Solid Edge part; units mm, degrees
sketch "Sketch1" plane through (0, 0, 0) normal (0, 0, 1) x (1, 0, 0)
  circle A0 centre (9.675, 10) radius 5
  circle A1 centre (9.675, 50) radius 5
  circle A2 centre (9.675, 90) radius 5
  circle A3 centre (70.325, 50) radius 5
  circle A4 centre (70.325, 90) radius 5
  circle A5 centre (70.325, 10) radius 5
  line L0 (0, 0) -> (80, 0)
  line L1 (80, 0) -> (80, 100)
  line L2 (0, 100) -> (80, 100)
  line L3 (0, 100) -> (0, 0)
extrude "Protrusion1" add sketch "Sketch1" along normal blind 10
sketch "Sketch2" plane through (40, 50, 10) normal (0, 0, 1) x (0, 1, 0)
  line L0 (-50, 20) -> (50, 20)
  line L1 (50, 20) -> (50, -20)
  line L2 (50, -20) -> (-50, -20)
  line L3 (-50, -20) -> (-50, 20)
extrude "ExtrudedProtrusion_2" add sketch "Sketch2" along normal blind 10
sketch "Sketch3" plane through (40, 50, 10) normal (0, 0, 1) x (0, 1, 0)
  circle A0 centre (0, 0) radius 12.5
extrude "ExtrudedCutout_1" cut sketch "Sketch3" along normal blind 10
sketch "Sketch4" plane through (40, 0, 10) normal (0, -1, 0) x (1, 0, 0)
  line L0 (20, 8) -> (20, 35)
  line L1 (-20, 35) -> (-20, 8)
  line L2 (-20, 8) -> (20, 8)
  arc A0 (-20, 35) -> (20, 35) centre (0, 35) cw
  circle A1 centre (0, 35) radius 10
extrude "ExtrudedCutout_6" cut sketch "Sketch4" against normal blind 10
sketch "Sketch5" plane through (40, 0, 10) normal (0, -1, 0) x (1, 0, 0)
  line L0 (20, 8) -> (20, 35)
  line L1 (-20, 35) -> (-20, 8)
  line L2 (-20, 8) -> (20, 8)
  arc A0 (-20, 35) -> (20, 35) centre (0, 35) cw
  circle A1 centre (0, 35) radius 10
extrude "ExtrudedProtrusion_3" add sketch "Sketch5" against normal blind 10
sketch "Sketch6" plane through (40, 0, 10) normal (0, -1, 0) x (1, 0, 0)
  circle A0 centre (0, 35) radius 17.5
  circle A1 centre (0, 35) radius 10
extrude "ExtrudedProtrusion_4" add sketch "Sketch6" along normal blind 3
mirror "Mirror1" about plane through (0, 50, 0) normal (0, -1, 0) of "ExtrudedProtrusion_3"
mirror "Mirror2" about plane through (0, 50, 0) normal (0, -1, 0) of "ExtrudedProtrusion_4"
sketch "Sketch7" plane through (40, 50, 10) normal (0, 0, 1) x (0, 1, 0)
  circle A0 centre (0, 0) radius 12.5
extrude "ExtrudedCutout_7" cut sketch "Sketch7" against normal blind 100
Work out the finished part from the listing and answer in its coordinate system (mm). A direction names the side the tool comes from. Give positions to 0.01 mm unless a question says otherwise; leave off trailing zeros. Loops run counter-clockwise (first coordinate to the right, second up) from the corner with the lowest first, then second, coordinate; pieces in that order, holes last. Notation, with made-up numbers: M 69.25,66 L 78.25,66 A22 cw 78.25,101 Z; hole C -21,10.25 d11. An arc over 180 degrees is marked long. One line per item, written item: value. Start each with the question number.
1. Determine the mould class of faces 5 (the face through (8.59, 94.88, 4.93)), 6 (the face through (32, 103, 53)), 7 (the face through (40, 5, 65)) for opening direction Y: released by +Y, released by -Y, zero draft, split by the parting line, or undercut.
2. Find section D-D (z = 58.5). Give the vertices of the cut face in (x, y), and give its area (3 significant figures).
3. Find section B-B (x = 40). Give the vertices of the cut face in (y, z).
4. Which of the six approach directions +Z, -Z, +X, -X, +Y, -Y give full straight-line access (tool end or side, diameter ignored) to faces 1 (the face through (40, 90, 32)), 2 (the face through (56.69, 101.48, 50.26)), 3 (the face through (17, 51, 10)), 4 (the face through (49.408, -1.479, 30.244))?
5. Each of these flat-tipped pins is pushed along its axis until it touches: P1, Ø6, axis at x = 70.325, y = 10, coming from the -Z side; P2, Ø3, axis at x = 30, y = 43, coming from the +Z side; P3, Ø22, axis at x = 73.5, y = 46.5, coming from the +Z side; P4, Ø5, axis at y = 26, z = 21.5, coming from the +X side. Where does it stop, or does it pass through?
6. Find the intervals of material crossed by probe 1 along Z at (x, y) = (40, 6); probe 2 along Y at (x, z) = (32, 55); probe 3 along Z at (x, y) = (72, 27), in increasing order.
7. Find section C-C (y = 17). Give the vertices of the cut face in (x, z).
8. Find section A-A (y = 50). Give the vertices of the cut face in (x, z) (3 decimals), and give its area (3 significant figures).
Reported:
1. face 5: undercut
1. face 6: released by +Y
1. face 7: zero draft
2. outline: M 25.24,0 L 28.86,0 L 28.86,-3 L 51.14,-3 L 51.14,0 L 54.76,0 L 54.76,10 L 25.24,10 Z; M 25.24,90 L 54.76,90 L 54.76,100 L 51.14,100 L 51.14,103 L 28.86,103 L 28.86,100 L 25.24,100 Z
2. area: 724 mm²
3. outline: M -3,27.5 L 0,27.5 L 0,0 L 37.5,0 L 37.5,20 L 10,20 L 10,35 L -3,35 Z; M -3,55 L 10,55 L 10,65 L 0,65 L 0,62.5 L -3,62.5 Z; M 62.5,0 L 100,0 L 100,27.5 L 103,27.5 L 103,35 L 90,35 L 90,20 L 62.5,20 Z; M 90,55 L 103,55 L 103,62.5 L 100,62.5 L 100,65 L 90,65 Z
4. face 1: +Z, +X, -X
4. face 2: +Y
4. face 3: +Z, -X, +Y, -Y
4. face 4: -Y
5. P1: passes through
5. P2: stops at z = 20
5. P3: stops at z = 10
5. P4: stops at x = 60
6. probe 1: z = 0 to 35, 55 to 65
6. probe 2: y = -3 to 10, 90 to 103
6. probe 3: z = 0 to 10
7. outline: M 0,0 L 80,0 L 80,10 L 60,10 L 60,20 L 20,20 L 20,10 L 0,10 Z
8. outline: M 0,0 L 4.675,0 L 4.675,10 L 0,10 Z; M 14.675,0 L 27.5,0 L 27.5,20 L 20,20 L 20,10 L 14.675,10 Z; M 52.5,0 L 65.325,0 L 65.325,10 L 60,10 L 60,20 L 52.5,20 Z; M 75.325,0 L 80,0 L 80,10 L 75.325,10 Z
8. area: 500 mm²
